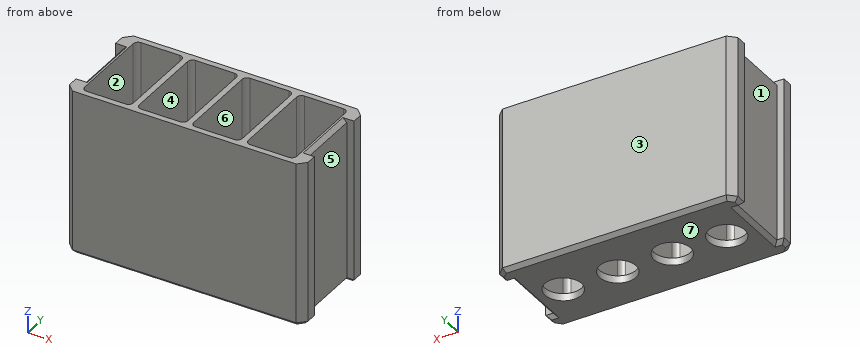
```python
from build123d import *

# Parameters (mm, degrees)
SKETCH1_W           = 92
SKETCH1_H           = 41.8
SKETCH1_W_2         = 20
SKETCH1_H_2         = 37
BOSS_EXTRUDE1_DEPTH = 65
SKETCH2_W           = 92
SKETCH2_H           = 41.8
BOSS_EXTRUDE2_DEPTH = 3
BOSS_EXTRUDE3_DEPTH = 68
CHAMFER4_SIZE       = 1.6
SKETCH3_R           = 7.5
CUT_EXTRUDE1_DEPTH  = 4
FILLET1_R           = 2
FILLET2_R           = 2
CHAMFER5_SIZE       = 1.6


with BuildPart() as part:
    # Sketch1 → Boss-Extrude1 (new body)
    with BuildSketch(Plane.XY):
        with Locations((33.6, 0)):
            Rectangle(SKETCH1_W, SKETCH1_H)
        with Locations((22.4, 0)):
            Rectangle(SKETCH1_W_2, SKETCH1_H_2, mode=Mode.SUBTRACT)
        Rectangle(SKETCH1_W_2, SKETCH1_H_2, mode=Mode.SUBTRACT)
        with Locations((44.8, 0)):
            Rectangle(SKETCH1_W_2, SKETCH1_H_2, mode=Mode.SUBTRACT)
        with Locations((67.2, 0)):
            Rectangle(SKETCH1_W_2, SKETCH1_H_2, mode=Mode.SUBTRACT)
    extrude(amount=BOSS_EXTRUDE1_DEPTH)

    # Sketch2 → Boss-Extrude2 (add)
    with BuildSketch(Plane(origin=(0, 0, 0), x_dir=(-1, 0, 0), z_dir=(0, 0, -1))):
        with Locations((-33.6, 0)):
            Rectangle(SKETCH2_W, SKETCH2_H)
    extrude(amount=BOSS_EXTRUDE2_DEPTH)

    # Sketch4 → Boss-Extrude3 (add)
    with BuildSketch(Plane(origin=(0, 0, -3), x_dir=(-1, 0, 0), z_dir=(0, 0, -1))):
        Polygon((-79.6, 20.9), (-79.6, 13.5), (-82.6, 13.5), (-82.6, 17.9), align=None)
        Polygon((-82.6, -13.5), (-82.6, -17.9), (-79.6, -20.9), (-79.6, -13.5), align=None)
    boss_extrude3 = extrude(amount=-BOSS_EXTRUDE3_DEPTH)

    # Mirror1: Boss-Extrude3 across plane
    add(boss_extrude3.mirror(Plane.ZY.offset(-33.6)))

    # Chamfer4
    chamfer4_edges = [part.edges().sort_by_distance(p)[0] for p in [
        (81.1, -13.5, -3),
        (82.6, -15.7, -3),
        (81.1, -19.4, -3),
        (-13.9, 19.4, -3),
        (-15.4, 15.7, -3),
        (-13.9, 13.5, -3),
        (-12.4, 0, -3),
        (-13.9, -13.5, -3),
        (-15.4, -15.7, -3),
        (-13.9, -19.4, -3),
        (33.6, 20.9, -3),
        (33.6, -20.9, -3),
        (79.6, 0, -3),
        (81.1, 19.4, -3),
        (82.6, 15.7, -3),
        (81.1, 13.5, -3),
    ]]
    chamfer(chamfer4_edges, length=CHAMFER4_SIZE)

    # Sketch3 → Cut-Extrude1 (cut, through all)
    with BuildSketch(Plane.XY):
        Circle(SKETCH3_R)
        with Locations((22.4, 0)):
            Circle(SKETCH3_R)
        with Locations((44.8, 0)):
            Circle(SKETCH3_R)
        with Locations((67.2, 0)):
            Circle(SKETCH3_R)
    extrude(amount=-CUT_EXTRUDE1_DEPTH, mode=Mode.SUBTRACT)

    # Fillet1
    fillet1_edges = [part.edges().sort_by_distance(p)[0] for p in [
        (10, -18.5, 32.5),
        (10, 18.5, 32.5),
        (-10, 18.5, 32.5),
        (-10, -18.5, 32.5),
        (32.4, 18.5, 32.5),
        (12.4, 18.5, 32.5),
        (12.4, -18.5, 32.5),
        (32.4, -18.5, 32.5),
        (54.8, 18.5, 32.5),
        (34.8, 18.5, 32.5),
        (34.8, -18.5, 32.5),
        (54.8, -18.5, 32.5),
        (77.2, 18.5, 32.5),
        (57.2, 18.5, 32.5),
        (57.2, -18.5, 32.5),
        (77.2, -18.5, 32.5),
    ]]
    fillet(fillet1_edges, radius=FILLET1_R)

    # Fillet2
    fillet2_edges = [part.edges().sort_by_distance(p)[0] for p in [
        (67.2, -18.5, 0),
        (77.2, 0, 0),
        (67.2, 18.5, 0),
        (57.2, 0, 0),
        (76.614213562, 17.914213562, 0),
        (57.785786438, 17.914213562, 0),
        (57.785786438, -17.914213562, 0),
        (76.614213562, -17.914213562, 0),
        (44.8, -18.5, 0),
        (54.8, 0, 0),
        (44.8, 18.5, 0),
        (34.8, 0, 0),
        (54.214213562, 17.914213562, 0),
        (35.385786438, 17.914213562, 0),
        (35.385786438, -17.914213562, 0),
        (54.214213562, -17.914213562, 0),
        (22.4, -18.5, 0),
        (32.4, 0, 0),
        (22.4, 18.5, 0),
        (12.4, 0, 0),
        (12.985786438, 17.914213562, 0),
        (31.814213562, 17.914213562, 0),
        (12.985786438, -17.914213562, 0),
        (31.814213562, -17.914213562, 0),
        (0, -18.5, 0),
        (10, 0, 0),
        (0, 18.5, 0),
        (-10, 0, 0),
        (-9.414213562, 17.914213562, 0),
        (9.414213562, 17.914213562, 0),
        (-9.414213562, -17.914213562, 0),
        (9.414213562, -17.914213562, 0),
    ]]
    fillet(fillet2_edges, radius=FILLET2_R)

    # Chamfer5
    chamfer5_edges = [part.edges().sort_by_distance(p)[0] for p in [
        (79.6, 0, 65),
        (-12.4, 0, 65),
    ]]
    chamfer(chamfer5_edges, length=CHAMFER5_SIZE)


solid = part.part
```
Geometry check sheet. Reference: the model listing, model coordinates, mm. Face numbers are marked on the shaded views. A direction names the side the tool comes from. Round coordinates to 2 decimals unless told otherwise and drop trailing zeros. Order: outer loops, then holes, each group sorted by start corner. A loop starts at its lowest first (then second) coordinate and runs counter-clockwise, first axis right, second up. Notation, with made-up numbers: (-40, 64.5) - (-18, 64.5) arc R23 ccw to (-18, 91.5) - close; hole circle Ø8 at (77.25, -33). An arc over 180 degrees is marked (long way). Use a Markdown table: item, result. Add a question column.
(1) Sectioned sample at D-D, the plane x = 21.5. Enter the section's corners in (y, z), and give its area (3 significant figures).
(2) Tool access check on the marked faces 5, 6 and 7. Record the directions out of +Z, -Z, +X, -X, +Y, -Y that give a thin tool (end or side, any length) a straight path to the whole face; none if there is none.
(3) Depth check by flat-ended pin: pin 1 (10 mm diameter, centred on x = 14.5, y = -2, fed in from +Z); pin 2 (9 mm diameter, centred on x = 67.2, y = 0, fed in from +Z); pin 3 (8 mm diameter, centred on y = 5.5, z = 15.5, fed in from +X); pin 4 (1.5 mm diameter, centred on x = 52.5, y = 5, fed in from +Z). Enter the tip coordinate at first touch or a pass-through.
(4) Sectioned sample at A-A, the plane x = 0. Enter the section's corners in (y, z).
(5) Sectioned sample at C-C, the plane y = -4.5. Count the separate pieces of the cut face and the enclosed holes in it, and give its area (3 significant figures).
(6) Release check for a two-part mould opening along X. For the marked faces 1, 2, 3 and 4 record: pulls with the +X half, pulls with the -X half, needs draft (parallel to the pull), parting line crosses it, or undercut.
(7) Material ranges on line 1 along X through (y, z) = (0, 31); line 2 along X through (y, z) = (-16.5, 5.5); line 3 along Y through (x, z) = (-5.5, 12.5), recorded low to high. Write a range as [from, to].
Answers below:
| question | item | result |
|---|---|---|
| 1 | outline | (-20.9, -1.4) - (-19.3, -3) - (-7.45, -3) - (-7.45, 0) - (-16.5, 0) arc R2 cw to (-18.5, 2) - (-18.5, 65) - (-20.9, 65) - close; (7.45, -3) - (19.3, -3) - (20.9, -1.4) - (20.9, 65) - (18.5, 65) - (18.5, 2) arc R2 cw to (16.5, 0) - (7.45, 0) - close |
| 1 | area | 392 mm² |
| 2 | face 5 | +Z, -Z, +X |
| 2 | face 6 | +Z |
| 2 | face 7 | -Z, +X, -X, +Y, -Y |
| 3 | pin 1 | z = 65 |
| 3 | pin 2 | through |
| 3 | pin 3 | x = 79.6 |
| 3 | pin 4 | z = 0.05 |
| 4 | outline | (-20.9, -1.4) - (-19.3, -3) - (-7.5, -3) - (-7.5, 0) - (-16.5, 0) arc R2 cw to (-18.5, 2) - (-18.5, 65) - (-20.9, 65) - close; (7.5, -3) - (19.3, -3) - (20.9, -1.4) - (20.9, 65) - (18.5, 65) - (18.5, 2) arc R2 cw to (16.5, 0) - (7.5, 0) - close |
| 5 | separate pieces | 5 |
| 5 | enclosed holes | 0 |
| 5 | area | 914 mm² |
| 6 | face 1 | pulls with the -X half |
| 6 | face 2 | undercut |
| 6 | face 3 | needs draft |
| 6 | face 4 | undercut |
| 7 | line 1 | [-12.4, -10], [10, 12.4], [32.4, 34.8], [54.8, 57.2], [77.2, 79.6] |
| 7 | line 2 | [-15.4, -10], [10, 12.4], [32.4, 34.8], [54.8, 57.2], [77.2, 82.6] |
| 7 | line 3 | [-20.9, -18.5], [18.5, 20.9] |
